Build history of the part. All positions in model axes, mm. Coordinates: 2 decimals unless noted, no trailing zeros. Loops run counter-clockwise (first coordinate to the right, second up) from the corner with the lowest first, then second, coordinate; pieces in that order, holes last.
Item 1: Cut at A-A (z = -0.3). List the corners of the cut face in (x, y), and give its area (3 significant figures).
Item 2: Cut at B-B (x = 417.5). List the corners of the cut face in (y, z), and give its area (3 significant figures).
Item 3: Drill centre lines: line 1 along Y through (x, z) = (299, -0.5); line 2 along X through (y, z) = (81, -0.15); line 3 along X through (y, z) = (54.5, -0.55) (3 decimals). Where is each one in solid material? Low to high.
from build123d import *

# Parameters (mm, degrees)
BRIDA_BASE1_DEPTH = 1.5875
REDONDEO2_R       = 20
REDONDEO3_R       = 50
REDONDEO4_R       = 20


# Sheet-metal steps are written as plain solids
with BuildPart() as part:
    # Croquis1 → Brida base1 (new body)
    with BuildSketch(Plane.XY):
        Polygon((-1104.973795497, 203.132185629), (178.706204503, 203.132185629), (178.706204503, 43.132185629), (547.966204503, 43.132185629), (547.966204503, -292.267814371), (-1104.973795497, -292.267814371), align=None)
    extrude(amount=-BRIDA_BASE1_DEPTH)

    # Redondeo2
    redondeo2_edges = [part.edges().sort_by_distance(p)[0] for p in [
        (178.706204503, 43.132185629, -0.79375),
    ]]
    fillet(redondeo2_edges, radius=REDONDEO2_R)

    # Redondeo3
    redondeo3_edges = [part.edges().sort_by_distance(p)[0] for p in [
        (178.706204503, 203.132185629, -0.79375),
    ]]
    fillet(redondeo3_edges, radius=REDONDEO3_R)

    # Redondeo4
    redondeo4_edges = [part.edges().sort_by_distance(p)[0] for p in [
        (547.966204503, 43.132185629, -0.79375),
    ]]
    fillet(redondeo4_edges, radius=REDONDEO4_R)


solid = part.part
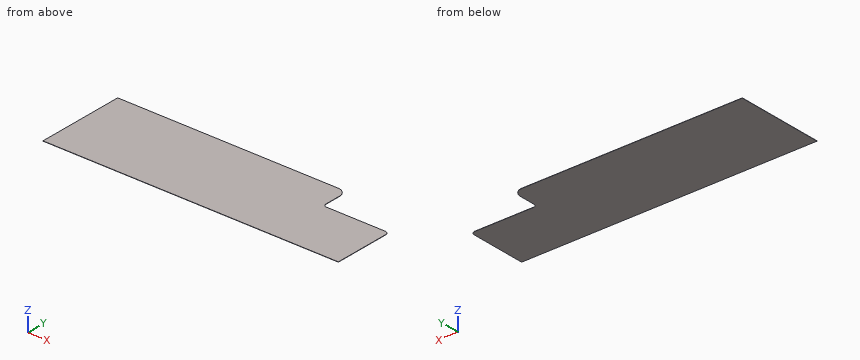
Filled sheet:
1. outline: (-1104.97, -292.27) - (547.97, -292.27) - (547.97, 23.13) arc R20 ccw to (527.97, 43.13) - (198.71, 43.13) arc R20 cw to (178.71, 63.13) - (178.71, 153.13) arc R50 ccw to (128.71, 203.13) - (-1104.97, 203.13) - close
1. area: 759,000 mm2
2. outline: (-292.27, -1.59) - (43.13, -1.59) - (43.13, 0) - (-292.27, 0) - close
2. area: 532 mm2
3. line 1: y = -292.27 to 43.13
3. line 2: x = -1104.97 to 178.71
3. line 3: x = -1104.974 to 180.665
